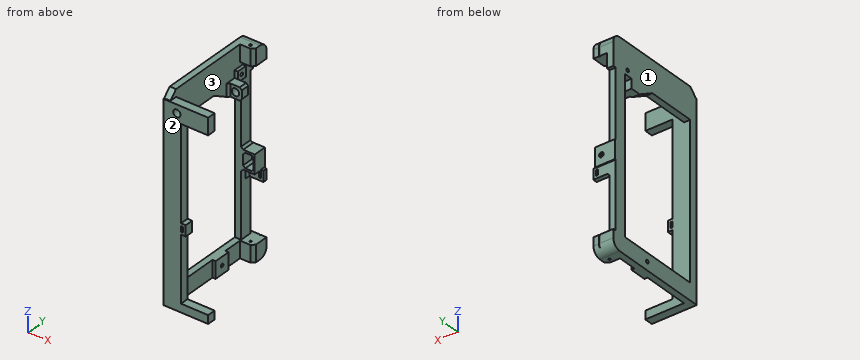
```python
from build123d import *
from build123d.topology import SkipClean

# Parameters (mm, degrees)
BOSS_EXTRUDE1_DEPTH             = 4
SKETCH2_W                       = 8
SKETCH2_H                       = 8
BOSS_EXTRUDE2_DEPTH             = 26
BOSS_EXTRUDE3_DEPTH             = 7
BOSS_EXTRUDE4_DEPTH             = 6
BOSS_EXTRUDE6_DEPTH             = 3
BOSS_EXTRUDE7_DEPTH             = 3
F_7_0MM_DOWEL_HOLE1_D           = 7
SKETCH6_W                       = 1.6
SKETCH6_H                       = 6
SKETCH9_W                       = 1.6
SKETCH9_H                       = 37
M3_CLEARANCE_HOLE4_D            = 3.2
BOSS_EXTRUDE8_DEPTH             = 8
BOSS_EXTRUDE9_DEPTH             = 6
SKETCH15_W                      = 12
SKETCH15_H                      = 8
BOSS_EXTRUDE10_DEPTH            = 13
CHAMFER1_SIZE                   = 2
CUT_EXTRUDE1_REACH              = 199.606
SKETCH16_R                      = 3.5
CHAMFER2_SIZE                   = 2
BOSS_EXTRUDE11_START            = 13
BOSS_EXTRUDE11_DEPTH            = 13
CUT_EXTRUDE2_DEPTH              = 218.195764231
CUT_EXTRUDE2_DEPTH_BACK         = 218.195764231
SKETCH18_R                      = 0.75
TAP_DRILL_FOR_M3X0_5_TAP1_D     = 2.5
TAP_DRILL_FOR_M3X0_5_TAP1_DEPTH = 16
F_2_0MM_DOWEL_HOLE4_D           = 2
CHAMFER3_SIZE                   = 3
BOSS_EXTRUDE12_START            = -13
SKETCH24_W                      = 18
SKETCH24_H                      = 12.6
BOSS_EXTRUDE12_DEPTH            = 19
SKETCH25_W                      = 14
SKETCH25_H                      = 11.1
CUT_EXTRUDE3_DEPTH              = 5
CHAMFER4_SIZE                   = 2
SKETCH26_W                      = 2.25
SKETCH26_H                      = 1.5
SKETCH27_W                      = 15.5
SKETCH27_H                      = 10.2
SKETCH27_W_2                    = 2
SKETCH27_H_2                    = 5.2
BOSS_EXTRUDE13_DEPTH            = 4
CHAMFER5_SIZE                   = 2
CHAMFER6_SIZE                   = 7


with BuildPart() as part:
    # Sketch1 → Boss-Extrude1 (new body)
    with BuildSketch(Plane(origin=(0, 0, 0), x_dir=(0, 0, -1), z_dir=(1, 0, 0))):
        Polygon((0, 0), (-8, 0), (-8, -8), (178, -8), (178, 0), (170, 0), align=None)
    extrude(amount=BOSS_EXTRUDE1_DEPTH)

    # Sketch2 → Boss-Extrude2 (add)
    with BuildSketch(Plane(origin=(4, 0, 0), x_dir=(0, 0, -1), z_dir=(1, 0, 0))):
        Polygon((-8, -8), (0, -8), (8, -8), (8, 0), (0, 0), (-8, 0), align=None)
        with Locations((174, -4)):
            Rectangle(SKETCH2_W, SKETCH2_H)
    extrude(amount=BOSS_EXTRUDE2_DEPTH)

    # Sketch1<2> → Boss-Extrude3 (add)
    with BuildSketch(Plane(origin=(0, 0, 0), x_dir=(0, 0, -1), z_dir=(1, 0, 0))):
        Polygon((0, 0), (-8, 0), (-8, -8), (178, -8), (178, 0), (170, 0), align=None)
    extrude(amount=-BOSS_EXTRUDE3_DEPTH)

    # Sketch4 → Boss-Extrude4 (add)
    with BuildSketch(Plane.ZY.offset(7)):
        with BuildLine():
            Line((-178, 0), (-178, 87))
            ThreePointArc((-178, 87), (-175.656854249, 92.656854249), (-170, 95))
            Line((-170, 95), (-162, 95))
            Line((-162, 95), (-162, 92))
            Line((-162, 92), (-15, 92))
            Line((-15, 92), (-15, 95))
            Line((-15, 95), (2.4, 95))
            Line((2.4, 95), (7, 95))
            ThreePointArc((7, 95), (12.656854249, 92.656854249), (15, 87))
            Line((15, 87), (15, 77.4))
            Line((15, 77.4), (15, 2.4))
            Line((15, 2.4), (15, 0))
            Line((15, 0), (8, 0))
            Line((8, 0), (8, -8))
            Line((8, -8), (-178, -8))
            Line((-178, -8), (-178, 0))
        make_face()
        Polygon((-15, 2.4), (-15, 0), (-162, 0), (-162, 80.4), (-15, 80.4), (-15, 77.4), align=None, mode=Mode.SUBTRACT)
    extrude(amount=BOSS_EXTRUDE4_DEPTH)

    # Sketch10 → Boss-Extrude6 (add)
    with BuildSketch(Plane(origin=(-7, 0, 0), x_dir=(0, 0, -1), z_dir=(1, 0, 0))):
        Polygon((15, 82.4), (5, 82.4), (5, 72.4), (10, 72.4), (15, 72.4), (15, 77.4), align=None)
    extrude(amount=BOSS_EXTRUDE6_DEPTH)

    # Sketch10<3> → Boss-Extrude7 (add)
    with BuildSketch(Plane(origin=(-7, 0, 0), x_dir=(0, 0, -1), z_dir=(1, 0, 0))):
        Polygon((170, 61), (178, 61), (178, 53), (178, 45), (162, 45), (162, 61), align=None)
    extrude(amount=BOSS_EXTRUDE7_DEPTH)

    # Ø7.0mm Dowel Hole1 (through all)
    with Locations(Plane.ZX):
        with Locations((0, 0)):
            Hole(F_7_0MM_DOWEL_HOLE1_D / 2)

    # Sketch6 → M3 Clearance Hole2 (revolve, cut)
    with BuildSketch(Plane(origin=(-7, 53, -170), x_dir=(0, 0, -1), z_dir=(0, 1, 0))):
        with Locations((0.8, 3)):
            Rectangle(SKETCH6_W, SKETCH6_H)
    revolve(axis=Axis((-0.65, 53, -170), (-1, 0, 0)), mode=Mode.SUBTRACT)

    # Sketch9 → M3 Clearance Hole3 (revolve, cut)
    with BuildSketch(Plane(origin=(-7, 77.4, -10), x_dir=(0, 0, 1), z_dir=(0, 1, 0))):
        with Locations((0.8, 18.5)):
            Rectangle(SKETCH9_W, SKETCH9_H)
    revolve(axis=Axis((-13.35, 77.4, -10), (1, 0, 0)), mode=Mode.SUBTRACT)

    # M3 Clearance Hole4 (through all)
    with Locations(Plane(origin=(0, 0, 0), x_dir=(0, 0, -1), z_dir=(1, 0, 0))):
        with Locations((10, 77.4), (170, 53)):
            Hole(M3_CLEARANCE_HOLE4_D / 2)

    # Sketch13 → Boss-Extrude8 (add)
    with BuildSketch(Plane(origin=(0, 0, 0), x_dir=(1, 0, 0), z_dir=(0, 1, 0))):
        Polygon((6, 107.7), (8.5, 107.7), (8.5, 97.5), (6, 97.5), (4, 97.5), (4, 100), (6, 100), (6, 105.2), (4, 105.2), (4, 107.7), align=None)
    extrude(amount=-BOSS_EXTRUDE8_DEPTH)

    # Sketch14 → Boss-Extrude9 (add)
    with BuildSketch(Plane(origin=(-7, 0, 0), x_dir=(0, 0, -1), z_dir=(1, 0, 0))):
        Polygon((15, 72.4), (24, 72.4), (24, 62.4), (15, 46.811542732), align=None)
    extrude(amount=-BOSS_EXTRUDE9_DEPTH)

    # Sketch15 → Boss-Extrude10 (add)
    with BuildSketch(Plane(origin=(-7, 0, 0), x_dir=(0, 0, -1), z_dir=(1, 0, 0))):
        with Locations((18, 68.4)):
            Rectangle(SKETCH15_W, SKETCH15_H)
    extrude(amount=BOSS_EXTRUDE10_DEPTH)

    # Chamfer1
    chamfer1_edges = [part.edges().sort_by_distance(p)[0] for p in [
        (-7, 64.4, -18),
    ]]
    chamfer(chamfer1_edges, length=CHAMFER1_SIZE)

    # Sketch16 → Cut-Extrude1 (cut, up to next)
    with BuildSketch(Plane(origin=(0, 72.4, 0), x_dir=(1, 0, 0), z_dir=(0, 1, 0)), mode=Mode.PRIVATE) as cut_extrude1_sk1:
        with Locations(Location((0, 18, 0), (0, 0, 270))):
            Circle(SKETCH16_R)
    cut_extrude1_tool1 = extrude(cut_extrude1_sk1.sketch, amount=-CUT_EXTRUDE1_REACH, mode=Mode.PRIVATE) & part.part
    add(cut_extrude1_tool1.solids().sort_by_distance((0, 72.4, -18))[0], mode=Mode.SUBTRACT)

    # Chamfer2
    chamfer2_edges = [part.edges().sort_by_distance(p)[0] for p in [
        (6, 68.4, -24),
        (6, 68.4, -12),
    ]]
    chamfer(chamfer2_edges, length=CHAMFER2_SIZE)

    # Sketch17 → Boss-Extrude11 (add)
    with BuildSketch(Plane(origin=(-7, 0, 0), x_dir=(0, 0, -1), z_dir=(1, 0, 0)).offset(BOSS_EXTRUDE11_START)):
        with BuildLine():
            Line((1, 95), (1, 79))
            Line((1, 79), (-15, 79))
            Line((-15, 79), (-15, 87))
            ThreePointArc((-15, 87), (-12.656854249, 92.656854249), (-7, 95))
            Line((-7, 95), (1, 95))
        make_face()
        with BuildLine():
            Line((170, 95), (162, 95))
            Line((162, 95), (162, 79))
            Line((162, 79), (178, 79))
            Line((178, 79), (178, 87))
            ThreePointArc((178, 87), (175.656854249, 92.656854249), (170, 95))
        make_face()
    extrude(amount=-BOSS_EXTRUDE11_DEPTH)

    # Sketch18 → Cut-Extrude2 (cut, two sides: drawn at the far end of the back side and taken through both)
    with BuildSketch(Plane.XY.offset(15).offset(-CUT_EXTRUDE2_DEPTH_BACK)):
        with Locations((0, 95)):
            Circle(SKETCH18_R)
    extrude(amount=CUT_EXTRUDE2_DEPTH + CUT_EXTRUDE2_DEPTH_BACK, mode=Mode.SUBTRACT)

    # Tap Drill for M3x0.5 Tap1
    with Locations(Plane(origin=(0, 83, 15), x_dir=(0, 1, 0), z_dir=(0, 0, 1))):
        with Locations((0, 0)):
            Hole(TAP_DRILL_FOR_M3X0_5_TAP1_D / 2, depth=TAP_DRILL_FOR_M3X0_5_TAP1_DEPTH)

    # Ø2.0mm Dowel Hole4 (through all)
    with Locations(Plane(origin=(0, 83, 15), x_dir=(0, 1, 0), z_dir=(0, 0, 1))):
        with Locations((0, 0)):
            Hole(F_2_0MM_DOWEL_HOLE4_D / 2)

    # Chamfer3
    chamfer3_edges = [part.edges().sort_by_distance(p)[0] for p in [
        (6, 79, 7),
        (6, 79, -170),
    ]]
    chamfer(chamfer3_edges, length=CHAMFER3_SIZE)

    # Sketch24 → Boss-Extrude12 (add)
    with SkipClean():  # the faces are left unmerged after this step: merging them gives an invalid solid
        with BuildSketch(Plane(origin=(0, 0, 0), x_dir=(0, 0, -1), z_dir=(1, 0, 0)).offset(BOSS_EXTRUDE12_START)):
            with Locations((89, 86.7)):
                Rectangle(SKETCH24_W, SKETCH24_H)
        extrude(amount=BOSS_EXTRUDE12_DEPTH)

    # Sketch25 → Cut-Extrude3 (cut, symmetric)
    with SkipClean():  # the faces are left unmerged after this step: merging them gives an invalid solid
        with BuildSketch(Plane(origin=(0, 0, 0), x_dir=(0, 0, -1), z_dir=(1, 0, 0))):
            with Locations((89, 85.95)):
                Rectangle(SKETCH25_W, SKETCH25_H)
        extrude(amount=CUT_EXTRUDE3_DEPTH, both=True, mode=Mode.SUBTRACT)

    # Chamfer4
    chamfer4_edges = [part.edges().sort_by_distance(p)[0] for p in [
        (-7, 86.2, -80),
        (-7, 86.2, -98),
        (-5, 85.95, -82),
        (-5, 85.95, -96),
        (5, 85.95, -82),
        (5, 85.95, -96),
    ]]
    chamfer(chamfer4_edges, length=CHAMFER4_SIZE)

    # Sketch26 → Cut-Revolve1 (revolve, cut)
    with SkipClean():  # the faces are left unmerged after this step: merging them gives an invalid solid
        with BuildSketch(Plane(origin=(0, 0, 0), x_dir=(0, 0, -1), z_dir=(1, 0, 0)), mode=Mode.PRIVATE) as cut_revolve1_sk:
            with Locations((87.875, 92.25)):
                Rectangle(SKETCH26_W, SKETCH26_H)
        revolve(cut_revolve1_sk.sketch.rotate(Axis((0, 65.518758018, -89), (0, 1, 0)), 180), axis=Axis((0, 65.518758018, -89), (0, 1, 0)), mode=Mode.SUBTRACT)

    # Sketch27 → Boss-Extrude13 (add)
    with SkipClean():  # the faces are left unmerged after this step: merging them gives an invalid solid
        with BuildSketch(Plane(origin=(0, 92, 0), x_dir=(1, 0, 0), z_dir=(0, 1, 0))):
            with Locations((0.75, 102.6)):
                Rectangle(SKETCH27_W, SKETCH27_H)
            with Locations((5, 102.6)):
                Rectangle(SKETCH27_W_2, SKETCH27_H_2, mode=Mode.SUBTRACT)
        extrude(amount=-BOSS_EXTRUDE13_DEPTH)

    # Chamfer5
    chamfer5_edges = [part.edges().sort_by_distance(p)[0] for p in [
        (-6, 88, -99),
        (-7, 88, -103.85),
        (-7, 90, -107.7),
        (0.5, 88, -98),
    ]]
    chamfer(chamfer5_edges, length=CHAMFER5_SIZE - 0.0001)  # a hair under: the kernel refuses the full size

    # Chamfer6
    chamfer6_edges = [part.edges().sort_by_distance(p)[0] for p in [
        (-10, 0, 8),
    ]]
    chamfer(chamfer6_edges, length=CHAMFER6_SIZE - 0.0001)  # a hair under: the kernel refuses the full size


solid = part.part
```
Check sheet for the modelled part. Datum: model origin and axes. Units: mm. Face numbers are marked on the shaded views. Give positions to 0.01 mm unless a question says otherwise; leave off trailing zeros. Order: outer loops, then holes, each group sorted by start corner. A loop starts at its lowest first (then second) coordinate and runs counter-clockwise, first axis right, second up. Notation, with made-up numbers: M -1.75,56 L 56.25,56 A22 cw 56.25,69 Z; hole C 29,-9 d9. An arc over 180 degrees is marked long. Answer in a Markdown table with one row per item. Add a question column.
Q1. Sectioned sample at D-D, the plane z = -18. Record the boundary of the cut face in (x, y), and give its area (3 significant figures).
Q2. Sectioned sample at A-A, the plane z = -89. Record the boundary of the cut face in (x, y), and give its area (3 significant figures).
Q3. Thickness scan on L1, parallel to X at y = 83, z = 8; L2, parallel to X at y = -4.5, z = 0; L3, parallel to Y at x = -4, z = -102. Record the ranges inside material, lowest first.
Q4. Sectioned sample at B-B, the plane y = 13.5. Record the boundary of the cut face in (x, z).
Q5. Sectioned sample at C-C, the plane x = 12. Record the boundary of the cut face in (y, z), and give its area (3 significant figures).
Q6. Gauge pin test, flat ends, axial feed: pin 1 Ø2.5 at (x, z) = (0, -89) entering from +Y; pin 2 Ø12 at (y, z) = (3, -117) entering from +X; pin 3 Ø1.6 at (x, y) = (4.5, 90) entering from +Z. Record the tip position at first contact, or that the pin passes through.
Q7. Release check for a two-part mould opening along Y. For the marked faces 1, 2 and 3 record: released by +Y, released by -Y, zero draft, split by the parting line, or undercut.
Verdict:
| question | item | result |
|---|---|---|
| 1 | outline | M -13,-8 L 4,-8 L 4,0 L -13,0 Z; M -13,52.01 L -7,52.01 L -7,62.4 L -5,64.4 L -3.5,64.4 L -3.5,72.4 L -13,72.4 Z; M -13,80.4 L -7,80.4 L -7,92 L -13,92 Z; M 3.5,64.4 L 6,64.4 L 6,72.4 L 3.5,72.4 Z |
| 1 | area | 378 mm² |
| 2 | outline | M -13,-8 L 4,-8 L 4,0 L -13,0 Z; M -13,80.4 L -5,80.4 L -5,91.5 L -2.25,91.5 L -2.25,93 L -13,93 Z; M 2.25,91.5 L 5,91.5 L 5,80.4 L 6,80.4 L 6,93 L 2.25,93 Z |
| 2 | area | 258 mm² |
| 3 | L1 | -13 to -1.25, 1.25 to 6 |
| 3 | L2 | -13 to -3.5, 3.5 to 30 |
| 3 | L3 | -8 to 0, 88 to 92 |
| 4 | outline | M -13,-178 L -7,-178 L -7,-162 L -13,-162 Z; M -13,-15 L -7,-15 L -7,15 L -13,15 Z |
| 5 | outline | M -8,-178 L 0,-178 L 0,-170 L -8,-170 Z; M -8,-8 L 0,-8 L 0,8 L -8,8 Z |
| 5 | area | 192 mm² |
| 6 | pin 1 | y = 0 |
| 6 | pin 2 | x = 4 |
| 6 | pin 3 | z = 14.69 |
| 7 | face 1 | zero draft |
| 7 | face 2 | released by -Y |
| 7 | face 3 | undercut |
